The model under review builds one solid part; all positions refer to its coordinate system, in mm. Face numbers are marked on the shaded views. Coordinates: 2 decimals unless noted, no trailing zeros. Loops run counter-clockwise (first coordinate to the right, second up) from the corner with the lowest first, then second, coordinate; pieces in that order, holes last. Notation, with made-up numbers: M 39.25,45 L 97.25,45 A28 ccw 97.25,73 Z; hole C 72,45.25 d7. An arc over 180 degrees is marked long. Write item = value, one per line. Start each with the question number.
Q1. Wall thickness on probe 1 along Y at (x, z) = (8, 0); probe 2 along Y at (x, z) = (2.5, -1.5); probe 3 along Z at (x, y) = (11.5, 1.25): over which ranges is each line inside the solid? List them lowest first.
Q2. We need section A-A on x = 4.25. Give the boundary of the cut face in (y, z), and give its area (3 significant figures).
Q3. Mouldability with a two-part tool opening along Y and no side actions: class the marked faces 1, 2 and 3 as released by +Y, released by -Y, zero draft, split by the parting line, or undercut.
Q4. Clearance check with flat-ended pins moving along their axes: pin 1 Ø0.6 at (x, z) = (-1, 0) entering from -Y; pin 2 Ø2 at (x, y) = (2, -2.5) entering from -Z. State where each tip first meets the part, or that it passes through.
Autodesk Inventor part; units mm, degrees
ref_plane "Work Plane1" through (29, 0, 0) normal (0, -1, 0) x (1, 0, 0)
ref_plane "YZ Plane" through (0, 0, 0) normal (1, 0, 0) x (0, 1, 0)
ref_plane "XZ Plane" through (0, 0, 0) normal (0, 1, 0) x (-1, 0, 0)
sketch "Sketch1" plane through (0, 0, 0) normal (0, 0, 1) x (1, 0, 0)
  line L0 (-0.0762, 0) -> (15.875, 0)
  line L1 (15.875, 0) -> (15.875, 1.7526)
  line L2 (15.875, 1.7526) -> (1.5902, 1.7526)
  line L3 (1.5902, 1.7526) -> (0.0001, 1.7526)
  line L4 (0.0001, 1.7526) -> (0, 1.7526)
  line L5 (0, 1.7526) -> (0, 3.3274)
  line L6 (0, 3.3274) -> (-1.8542, 3.3274)
  line L7 (-1.8542, 3.3274) -> (-1.8542, 1.1438)
  line L8 (-1.8542, 1.1438) -> (-0.7366, 1.1438)
  line L9 (-0.7366, 1.1438) -> (-0.0762, 0)
  line L10 (-5.4, 0) -> (19.4208, 0)
  line L11 (0, -0.6655) -> (0, 3.9929)
  line L12 (1.5902, 1.7526) -> (0, 1.7526) construction
  dimension "d1" = 14.2848
  dimension "d2" = 1.5901
  dimension "d3" = 1.8542
  dimension "d4" = 1.1176
  dimension "d5" = 60
  dimension "d6" = 3.5052
  dimension "d7" = 3.5052
  dimension "d8" = 2.2877
  dimension "d9" = 6.6548
  dimension "d26" = 15.875
revolve "Body" add sketch "Sketch1" angle 360 about axis through (-0.0762, 0, 0) along (1, 0, 0)
sketch "Sketch2" plane through (-1.8542, 0, 0) normal (-1, 0, 0) x (0, 0, 1)
  circle A0 centre (0, 0) radius 1.1438
  line L0 (0, -4.6584) -> (0, 4.6584)
  line L1 (-4.6584, 0) -> (4.6584, 0)
  line L2 (1.1438, 0) -> (0.5719, -0.9906)
  line L3 (0.5719, -0.9906) -> (-0.5719, -0.9906)
  line L4 (-0.5719, -0.9906) -> (-1.1438, 0)
  line L5 (-1.1438, 0) -> (-0.5719, 0.9906)
  line L6 (-0.5719, 0.9906) -> (0.5719, 0.9906)
  line L7 (0.5719, 0.9906) -> (1.1438, 0)
extrude "Slot" add sketch "Sketch2" against normal up to next contours L7 A0 | A0 L2 | L6 L0 A0 | A0 L0 L3 | L0 L6 A0 | A0 L3 L0 | L4 A0 | A0 L5
fillet "Fillet1" radius 1.6002 1 edges at (-1.8542, -3.3274, 0)
thread "Thread"
chamfer "Chamfer1" distance 0.4869 distance2 0.4869 1 edges at (15.875, -1.7526, 0) measured on face at (15.875, -0.5973, -0.3874)
ref_plane "Work Plane1" through (29, 0, 0) normal (0, -1, 0) x (1, 0, 0)
fillet "Fillet2" radius 0.1 1 edges at (0.0001, -1.7526, 0)
equation "\"d1\" = GEL"
equation "\"d3\" = KOH"
equation "\"d4\" = INTI"
equation "\"d6\" = GD"
equation "\"d7\" = BDM"
equation "\"d8\" = 1.1547 * SW"
equation "\"d9\" = KOD"
equation "\"d26\" = NLG"
equation "\"d30\" = R"
equation "\"d17\" = RR"
equation "\"d13\" = GEL"
equation "\"d15\" = -0.5 * SPD + 0.5 * GD"
equation "\"d16\" = GUL"
equation "\"GD\" = NND"
equation "\"NLG\" = 15.875"
equation "\"GEL\" = 14.28476"
equation "\"KOD\" = 6.6548"
equation "\"KOH\" = 1.8542"
equation "\"INTI\" = 1.1176"
equation "\"GAL\" = 1.59004"
equation "\"GUL\" = 0.48692"
equation "\"BDM\" = NND"
equation "\"SW\" = 1.9812"
equation "\"RR\" = 1.6002"
equation "\"SPD\" = 2.53136"
equation "\"R\" = 0.1"
equation "\"TOA\" = 30deg"
equation "\"GD1\" = SPD"
equation "\"THREADDIA\" = 3.5052"
equation "\"KOH1\" = 0.381"
equation "\"NND\" = 3.5052"
equation "\"E0\" = 2.28829"
properties part number "ANSI B18.3 - 6 - 32 x 5/8" material "Steel, Mild"
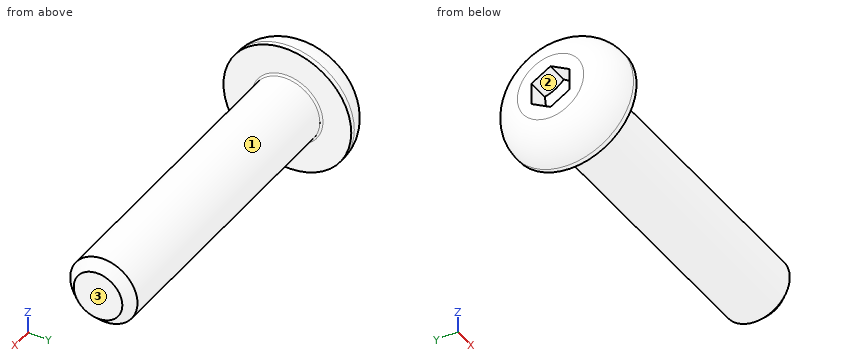
Returned:
q1.probe_1 = -1.75 to 1.75
q1.probe_2 = -0.91 to 0.91
q1.probe_3 = -1.23 to 1.23
q2.outline = C 0,0 d3.51
q2.area = 9.65 mm^2
q3.face_1 = split by the parting line
q3.face_2 = undercut
q3.face_3 = zero draft
q4.pin_1 = -3.26
q4.pin_2 = -0.91
